from build123d import *

# Parameters (mm, degrees)
SKETCH_1_R          = 42
SKETCH_1_R_2        = 3.1
EXTRUDE_1_DEPTH     = 6
SKETCH_2_R          = 29
CUT_EXTRUDE_1_DEPTH = 1
FILLET_3_R          = 1
SKETCH_3_R          = 29
SKETCH_3_R_2        = 23.5
EXTRUDE_2_DEPTH     = 8.3
CHAMFER_1_SIZE      = 1
SKETCH_4_R          = 12.5
CUT_EXTRUDE_2_DEPTH = 8.3


with BuildPart() as part:
    # Эскиз1 → Бобышка-Вытянуть1 (new body)
    with BuildSketch(Plane.XY):
        Circle(SKETCH_1_R)
        with Locations((0, 36)):
            Circle(SKETCH_1_R_2, mode=Mode.SUBTRACT)
        with Locations((36, 0)):
            Circle(SKETCH_1_R_2, mode=Mode.SUBTRACT)
        with Locations((0, -36)):
            Circle(SKETCH_1_R_2, mode=Mode.SUBTRACT)
        with Locations((-36, 0)):
            Circle(SKETCH_1_R_2, mode=Mode.SUBTRACT)
    extrude(amount=EXTRUDE_1_DEPTH)

    # Эскиз2 → Вырез-Вытянуть1 (cut)
    with BuildSketch(Plane.XY.offset(6)):
        Circle(SKETCH_2_R)
    extrude(amount=-CUT_EXTRUDE_1_DEPTH, mode=Mode.SUBTRACT)

    # Скругление3
    fillet_3_edges = [part.edges().sort_by_distance(p)[0] for p in [
        (-29, 0, 5),
    ]]
    fillet(fillet_3_edges, radius=FILLET_3_R - 0.0001)  # a hair under: the kernel refuses the full size

    # Эскиз3 → Бобышка-Вытянуть2 (add)
    with BuildSketch(Plane(origin=(0, 0, 0), x_dir=(-1, 0, 0), z_dir=(0, 0, -1))):
        with Locations(Location((0, 0, 0), (0, 0, 180))):
            Circle(SKETCH_3_R)
        with Locations(Location((0, 0, 0), (0, 0, 180))):
            Circle(SKETCH_3_R_2, mode=Mode.SUBTRACT)
    extrude(amount=EXTRUDE_2_DEPTH)

    # Фаска1
    chamfer_1_edges = [part.edges().sort_by_distance(p)[0] for p in [
        (-23.5, 0, 0),
    ]]
    chamfer(chamfer_1_edges, length=CHAMFER_1_SIZE)

    # Эскиз4 → Вырез-Вытянуть2 (cut)
    with BuildSketch(Plane(origin=(0, 0, 0), x_dir=(-1, 0, 0), z_dir=(0, 0, -1))):
        Circle(SKETCH_4_R)
    extrude(amount=-CUT_EXTRUDE_2_DEPTH, mode=Mode.SUBTRACT)


solid = part.part
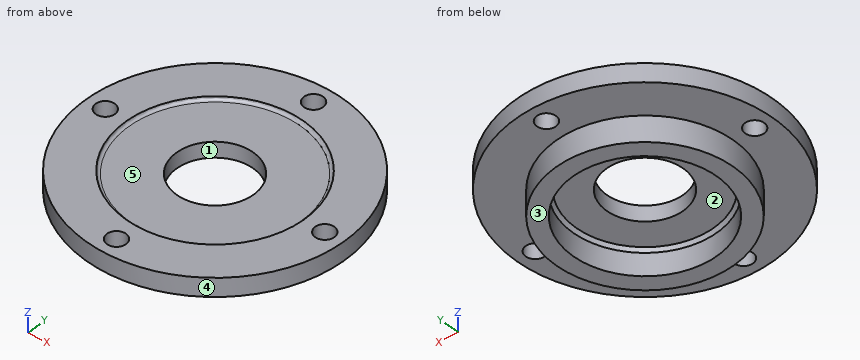
Design review of the part built by this model. Coordinates are the model's own, in mm. Face numbers are marked on the shaded views. A direction names the side the tool comes from. Coordinates: 2 decimals unless noted, no trailing zeros. Order: outer loops, then holes, each group sorted by start corner. A loop starts at its lowest first (then second) coordinate and runs counter-clockwise, first axis right, second up. Notation, with made-up numbers: (9, 80.25) -> (54, 80.25) arc R11 cw to (54, 89.25) -> close; hole circle Ø1 at (46.25, -11.75). An arc over 180 degrees is marked (long way). Use one line per item in the form item = value. Start each with the question number.
(1) Add section C-C on y = 34.5. State the section outline as (x, z) points.
(2) Insertion check: pin 1 (4 mm diameter, centred on x = 2, z = -1.5, fed in from -Y); pin 2 (22.5 mm diameter, centred on x = -4.5, y = -1, fed in from -Z); pin 3 (3 mm diameter, centred on x = 14, y = 20, fed in from +Z); pin 4 (10 mm diameter, centred on x = -22, y = -7, fed in from -Z). Each pin has a flat end and moves straight along its axis. Give the tip position at first contact, or say it passes through.
(3) For probe 1 along Y at (x, z) = (0, 1.7); probe 2 along Z at (x, y) = (29, -18); probe 3 along Y at (x, z) = (-36, 4.05), list the stretches that pass through material, from the lowest coordinate up.
(4) For the marked faces 1 and 2, list the 3-axis set-ups (+Z, -Z, +X, -X, +Y, -Y) from which the entire face can be reached by the end or side of a thin tool; tool diameter is ignored.
(5) Add section D-D on z = 2.75. State the section outline as (x, y) points, plus the area to 3 significant figures.
(6) The part is to be moulded in two halves that separate along Y. For the marked faces 3, 4 and 5, say which applies: +Y half, -Y half, draft (parallel to the pull), parting line (faces both ways), or undercut.
(7) Add section A-A on x = 0. Give the number of separate pieces and of enclosed holes in the cut face, plus the area to 3 significant figures.
Answer block:
q1.outline = (-23.95, 0) -> (-2.71, 0) -> (-2.71, 6) -> (-23.95, 6) -> close; (2.71, 0) -> (23.95, 0) -> (23.95, 6) -> (2.71, 6) -> close
q2.pin_1 = -41.99
q2.pin_2 = 0
q2.pin_3 = 5
q2.pin_4 = -8.3
q3.probe_1 = -42 to -39.1, -32.9 to -12.5, 12.5 to 32.9, 39.1 to 42
q3.probe_2 = 0 to 6
q3.probe_3 = -21.63 to -3.1, 3.1 to 21.63
q4.face_1 = +Z, -Z
q4.face_2 = -Z
q5.outline = circle Ø84 at (0, 0); hole circle Ø6.2 at (-36, 0); hole circle Ø25 at (0, 0); hole circle Ø6.2 at (0, -36); hole circle Ø6.2 at (0, 36); hole circle Ø6.2 at (36, 0)
q5.area = 4,930 mm²
q6.face_3 = draft
q6.face_4 = parting line
q6.face_5 = undercut
q7.separate_pieces = 4
q7.enclosed_holes = 0
q7.area = 339 mm²
